Source: CAD feature listing. Evaluate the final solid. Frame: model axes, mm. A direction names the side the tool comes from. Give positions to 0.01 mm unless a question says otherwise; leave off trailing zeros. Loops run counter-clockwise (first coordinate to the right, second up) from the corner with the lowest first, then second, coordinate; pieces in that order, holes last. Notation, with made-up numbers: M 15.25,-31 L 46.25,-31 A8 cw 46.25,-23 Z; hole C 29.25,54.25 d8. An arc over 180 degrees is marked long. Answer in a Markdown table with one row per item.
```python
from build123d import *

# Parameters (mm, degrees)
SKETCH1_R               = 60
BOSS_EXTRUDE1_DEPTH     = 33.6
CUT_EXTRUDE2_DEPTH      = 92.263136041
CUT_EXTRUDE2_DEPTH_BACK = 92.263136041
SKETCH2_R               = 2
SKETCH4_R               = 24.5
CUT_EXTRUDE3_DEPTH      = 5
SKETCH5_R               = 42.5
BOSS_EXTRUDE2_DEPTH     = 11.5
CUT_EXTRUDE4_DEPTH      = 97.093756301
CUT_EXTRUDE4_DEPTH_BACK = 11.5


with BuildPart() as part:
    # Sketch1 → Boss-Extrude1 (new body)
    with BuildSketch(Plane(origin=(0, 0, 0), x_dir=(1, 0, 0), z_dir=(0, 1, 0))):
        with Locations(Location((0, 0, 0), (0, 0, 270))):
            Circle(SKETCH1_R)
    extrude(amount=BOSS_EXTRUDE1_DEPTH)

    # Sketch2 → Cut-Extrude2 (cut, two sides: drawn at the far end of the back side and taken through both)
    with BuildSketch(Plane(origin=(0, 33.6, 0), x_dir=(1, 0, 0), z_dir=(0, 1, 0)).offset(-CUT_EXTRUDE2_DEPTH_BACK)):
        with Locations(Location((0, 53, 0), (0, 0, 270))):
            Circle(SKETCH2_R)
        with Locations(Location((31.152618372, 42.877900702, 0), (0, 0, 270))):
            Circle(SKETCH2_R)
        with Locations(Location((50.405995364, 16.377900702, 0), (0, 0, 270))):
            Circle(SKETCH2_R)
        with Locations(Location((50.405995364, -16.377900702, 0), (0, 0, 270))):
            Circle(SKETCH2_R)
        with Locations(Location((31.152618372, -42.877900702, 0), (0, 0, 270))):
            Circle(SKETCH2_R)
        with Locations(Location((0, -53, 0), (0, 0, 270))):
            Circle(SKETCH2_R)
        with Locations(Location((-31.152618372, -42.877900702, 0), (0, 0, 270))):
            Circle(SKETCH2_R)
        with Locations(Location((-50.405995364, -16.377900702, 0), (0, 0, 270))):
            Circle(SKETCH2_R)
        with Locations(Location((-50.405995364, 16.377900702, 0), (0, 0, 270))):
            Circle(SKETCH2_R)
        with Locations(Location((-31.152618372, 42.877900702, 0), (0, 0, 270))):
            Circle(SKETCH2_R)
    extrude(amount=CUT_EXTRUDE2_DEPTH + CUT_EXTRUDE2_DEPTH_BACK, mode=Mode.SUBTRACT)

    # Sketch4 → Cut-Extrude3 (cut)
    with BuildSketch(Plane(origin=(0, 33.6, 0), x_dir=(1, 0, 0), z_dir=(0, 1, 0))):
        with Locations(Location((0, 0, 0), (0, 0, 270))):
            Circle(SKETCH4_R)
    extrude(amount=-CUT_EXTRUDE3_DEPTH, mode=Mode.SUBTRACT)

    # Sketch5 → Boss-Extrude2 (add)
    with BuildSketch(Plane.XZ):
        with Locations(Location((0, 0, 0), (0, 0, 90))):
            Circle(SKETCH5_R)
    extrude(amount=BOSS_EXTRUDE2_DEPTH)

    # Sketch6 → Cut-Extrude4 (cut, two sides: drawn at the far end of the back side and taken through both)
    with BuildSketch(Plane.XZ.offset(11.5).offset(-CUT_EXTRUDE4_DEPTH_BACK)):
        with BuildLine():
            Line((14.2, -40.057583552), (-14.2, -40.057583552))
            ThreePointArc((-14.2, -40.057583552), (0, -42.5), (14.2, -40.057583552))
        make_face()
    extrude(amount=CUT_EXTRUDE4_DEPTH + CUT_EXTRUDE4_DEPTH_BACK, mode=Mode.SUBTRACT)


solid = part.part
```
1) Section D-D, the plane y = 25. Count the separate pieces of the cut face and the enclosed holes in it, then the cut area to 3 significant figures.
Reply:
| item | result |
|---|---|
| separate pieces | 1 |
| enclosed holes | 10 |
| area | 11,200 mm² |
2) Set-up query: faces 4 (the cylindrical face through (7.36, 31.14, 23.37)), 5 (the cylindrical face through (1.666, -5.67, 42.467)), 6 (the flat face through (0, -6, -40.058)). Return all of +Z, -Z, +X, -X, +Y, -Y with unobstructed straight access to the full face (end or side cutting, diameter ignored); none if empty.
Reply:
| item | result |
|---|---|
| face 4 | +Y |
| face 5 | -Y |
| face 6 | -Z, +X, -X, -Y |
3) Material intervals for L1, parallel to X at y = 19, z = -17.5; L2, parallel to Y at x = 20.5, z = 11; L3, parallel to Y at x = -51.5, z = 10, sorted ascending.
Reply:
| item | result |
|---|---|
| L1 | x = -57.39 to -52.06, -48.75 to 48.75, 52.06 to 57.39 |
| L2 | y = -11.5 to 28.6 |
| L3 | y = 0 to 33.6 |
4) Section B-B, the plane z = 0. Return loops of the section in (x, y), then the cut area to 3 significant figures.
Reply:
| item | result |
|---|---|
| outline | M -60,0 L -42.5,0 L -42.5,-11.5 L 42.5,-11.5 L 42.5,0 L 60,0 L 60,33.6 L 24.5,33.6 L 24.5,28.6 L -24.5,28.6 L -24.5,33.6 L -60,33.6 Z |
| area | 4,760 mm² |
5) Pin query (flat end, axial travel): pin 1 Ø2 at (y, z) = (14.5, -19.5) entering from +X; pin 2 Ø8 at (y, z) = (1.5, -27.5) entering from +X; pin 3 Ø1.5 at (y, z) = (-5, -27) entering from +X. Return the tip coordinate at first contact, or that it passes through.
Reply:
| item | result |
|---|---|
| pin 1 | stops at x = 57.08 |
| pin 2 | stops at x = 55.21 |
| pin 3 | stops at x = 33.42 |
6) Section C-C, the plane z = 53. Return loops of the section in (x, y).
Reply:
| item | result |
|---|---|
| outline | M -28.12,0 L -2,0 L -2,33.6 L -28.12,33.6 Z; M 2,0 L 28.12,0 L 28.12,33.6 L 2,33.6 Z |
7) Pull-direction query (X, two-part tool) for faces 1 (the flat face through (1, 0, -41)), 2 (the cylindrical face through (2.64, 16.56, -59.94)), 3 (the cylindrical face through (-49.05, 16.56, -17.85)); classes: released by +X, released by -X, zero draft, split by the parting line, or undercut.
Reply:
| item | result |
|---|---|
| face 1 | zero draft |
| face 2 | split by the parting line |
| face 3 | undercut |
8) Section A-A, the plane x = 0. Return loops of the section in (y, z).
Reply:
| item | result |
|---|---|
| outline | M -11.5,-40.06 L 0,-40.06 L 0,-51 L 33.6,-51 L 33.6,-24.5 L 28.6,-24.5 L 28.6,24.5 L 33.6,24.5 L 33.6,51 L 0,51 L 0,42.5 L -11.5,42.5 Z; M 0,-60 L 33.6,-60 L 33.6,-55 L 0,-55 Z; M 0,55 L 33.6,55 L 33.6,60 L 0,60 Z |
